Design review of the part built by this model. Coordinates are the model's own, in mm. A direction names the side the tool comes from. Round coordinates to 2 decimals unless told otherwise and drop trailing zeros. Loops run counter-clockwise (first coordinate to the right, second up) from the corner with the lowest first, then second, coordinate; pieces in that order, holes last. Notation, with made-up numbers: (67, 58) -> (98, 58) arc R22 cw to (98, 78) -> close; hole circle Ø8 at (-31, 68.5). An arc over 180 degrees is marked (long way). Write each question's results on one line, items separated by ' | '. Start each with the question number.
from build123d import *

# Parameters (mm, degrees)
F1_DEPTH = 184.15
F2_W     = 124.7902
F2_H     = 174.5742
F3_DEPTH = 5.715
F5_DEPTH = 3.175


with BuildPart() as f1:
    # F0 (on Front) → F1 (new body)
    with BuildSketch(Plane.XZ):
        with BuildLine():
            Line((0, 2.641868), (0, 0))
            Line((0, 0), (133.35, 0))
            Line((133.35, 0), (133.35, 2.641868))
            ThreePointArc((133.35, 2.641868), (121.39739, 14.594478), (133.35, 26.547088))
            Line((133.35, 26.547088), (133.35, 29.188956))
            Line((133.35, 29.188956), (0, 29.188956))
            Line((0, 29.188956), (0, 26.547088))
            ThreePointArc((0, 26.547088), (11.95261, 14.594478), (0, 2.641868))
        make_face()
    extrude(amount=F1_DEPTH)

    # F2 (on face) → F3 (join)
    with BuildSketch(Plane.XY.offset(29.188956)):
        with Locations((66.9671, -91.8591)):
            Rectangle(F2_W, F2_H)
    extrude(amount=F3_DEPTH)

    # F4 (on face) → F5 (cut)
    with BuildSketch(Plane.XY.offset(34.903956)):
        Polygon((85.200642, -145.579033), (123.752596, -171.298692), (110.021826, -123.877873), align=None)
    extrude(amount=-F5_DEPTH, mode=Mode.SUBTRACT)


solid = f1.part
1) The part is to be moulded in two halves that separate along X. For faces 1 (the face through (4.572, -93, 32)), 2 (the face through (97.78, -134.58, 33.34)), 3 (the face through (131, -92, 29.189)), say which applies: +X half, -X half, draft (parallel to the pull), parting line (faces both ways), or undercut.
2) Take a section at B-B (x = 108). Write out the cut boundary in (y, z).
3) Insertion check: pin 1 (1.5 mm diameter, centred on y = -56.5, z = 30.5, fed in from -X); pin 2 (4.5 mm diameter, centred on x = 46, z = 33, fed in from +Y); pin 3 (3 mm diameter, centred on y = -157, z = 11, fed in from -X). Each pin has a flat end and moves straight along its axis. Give the tip position at first contact, or say it passes through.
4) To check wall thickness, follow line 1 (X direction, y = -15, z = 29.5); line 2 (Z direction, x = 118, y = -164.5); line 3 (Y direction, x = 45.5, z = 32.5). State the ranges of each line that lie inside material, in increasing order. Write a range as from..to.
5) Take a section at C-C (z = 19.5). Write out the cut boundary in (x, y), plus the area to 3 significant figures.
6) Take a section at D-D (y = -129.5). Write out the cut boundary in (x, z), plus the area to 3 significant figures.
7) Take a section at A-A (y = -149.5). Write out the cut boundary in (x, z), plus the area to 3 significant figures.
8) For faces 4 (the face through (66, -4.572, 32)), 5 (the face through (129.362, -93, 32)), 6 (the face through (108, -147, 31.729)), 7 (the face through (66, -179.146, 32)), list the 3-axis set-ups (+Z, -Z, +X, -X, +Y, -Y) from which the entire face can be reached by the end or side of a thin tool; tool diameter is ignored.
Geometry check:
1) face 1: -X half | face 2: undercut | face 3: draft
2) outline: (-184.15, 0) -> (0, 0) -> (0, 29.19) -> (-4.57, 29.19) -> (-4.57, 34.9) -> (-125.65, 34.9) -> (-125.65, 31.73) -> (-160.79, 31.73) -> (-160.79, 34.9) -> (-179.15, 34.9) -> (-179.15, 29.19) -> (-184.15, 29.19) -> close
3) pin 1: stops at x = 4.57 | pin 2: stops at y = -4.57 | pin 3: stops at x = 10.81
4) line 1: x = 4.57..129.36 | line 2: z = 0..31.73 | line 3: y = -179.15..-4.57
5) outline: (10.9, -184.15) -> (122.45, -184.15) -> (122.45, 0) -> (10.9, 0) -> close | area: 20,500 mm^2
6) outline: (0, 0) -> (133.35, 0) -> (133.35, 2.64) arc R11.95 cw to (133.35, 26.55) -> (133.35, 29.19) -> (129.36, 29.19) -> (129.36, 34.9) -> (111.65, 34.9) -> (111.65, 31.73) -> (103.59, 31.73) -> (103.59, 34.9) -> (4.57, 34.9) -> (4.57, 29.19) -> (0, 29.19) -> (0, 26.55) arc R11.95 cw to (0, 2.64) -> close | area: 4,130 mm^2
7) outline: (0, 0) -> (133.35, 0) -> (133.35, 2.64) arc R11.95 cw to (133.35, 26.55) -> (133.35, 29.19) -> (129.36, 29.19) -> (129.36, 34.9) -> (117.44, 34.9) -> (117.44, 31.73) -> (91.08, 31.73) -> (91.08, 34.9) -> (4.57, 34.9) -> (4.57, 29.19) -> (0, 29.19) -> (0, 26.55) arc R11.95 cw to (0, 2.64) -> close | area: 4,070 mm^2
8) face 4: +Z, +X, -X, +Y | face 5: +Z, +X, +Y, -Y | face 6: +Z | face 7: +Z, +X, -X, -Y
